Could you check a few things on this drawing? It's one solid part, dimensions in mm from its lowest x, y, z. A direction names the side the tool comes from. Give positions to 0.01 mm unless a question says otherwise; leave off trailing zeros. Write each loop counter-clockwise with the first axis right and the second up, starting at its lowest first coordinate (ties: lowest second). Pieces come first, ordered by that corner, then holes. Notation, with made-up numbers: (-1, 69.5) -> (26, 69.5) arc R23 ccw to (26, 78.5) -> close; hole circle Ø7 at (-25.5, 29). An arc over 180 degrees is marked (long way). Answer as CSV lines item,"result". Start each with the question number.
1. If we mould it in two halves opening along X, with no side actions, what happens to the marked faces 3, 4 and 5? For each: pulls with the +X half, pulls with the -X half, needs draft (parallel to the pull), parting line crosses it, or undercut.
2. I need wall thicknesses on line 1 (Y direction, x = 4.95, z = 11.15); line 2 (Z direction, x = 5.5, y = 3); line 3 (Z direction, x = 4.75, y = 2). Which ranges of each line are inside material? Lowest first, please. Write a range as [from, to].
3. If we section it at A-A on x = 4.95: Write out the boundary of the cut face in (y, z).
4. If we section it at D-D on y = 7.75: Write out the boundary of the cut face in (x, z).
5. On a 3-axis mill with a long thin cutter (end or side, diameter ignored), from which of +Z, -Z, +X, -X, +Y, -Y can I reach the whole of each face in a straight line? I mean the marked faces 1 and 2. Say none if no direction works.
6. I'm going to push flat-ended pins straight in: P1, Ø1.8, axis at x = 1.45, y = 4.95, coming from the +Z side; P2, Ø2, axis at y = 8, z = 3, coming from the -X side; P3, Ø2, axis at x = 2, z = 6, coming from the -Y side. Where does each tip first touch, or does it pass through?
7. If we section it at C-C on z = 14: Write out the boundary of the cut face in (x, y).
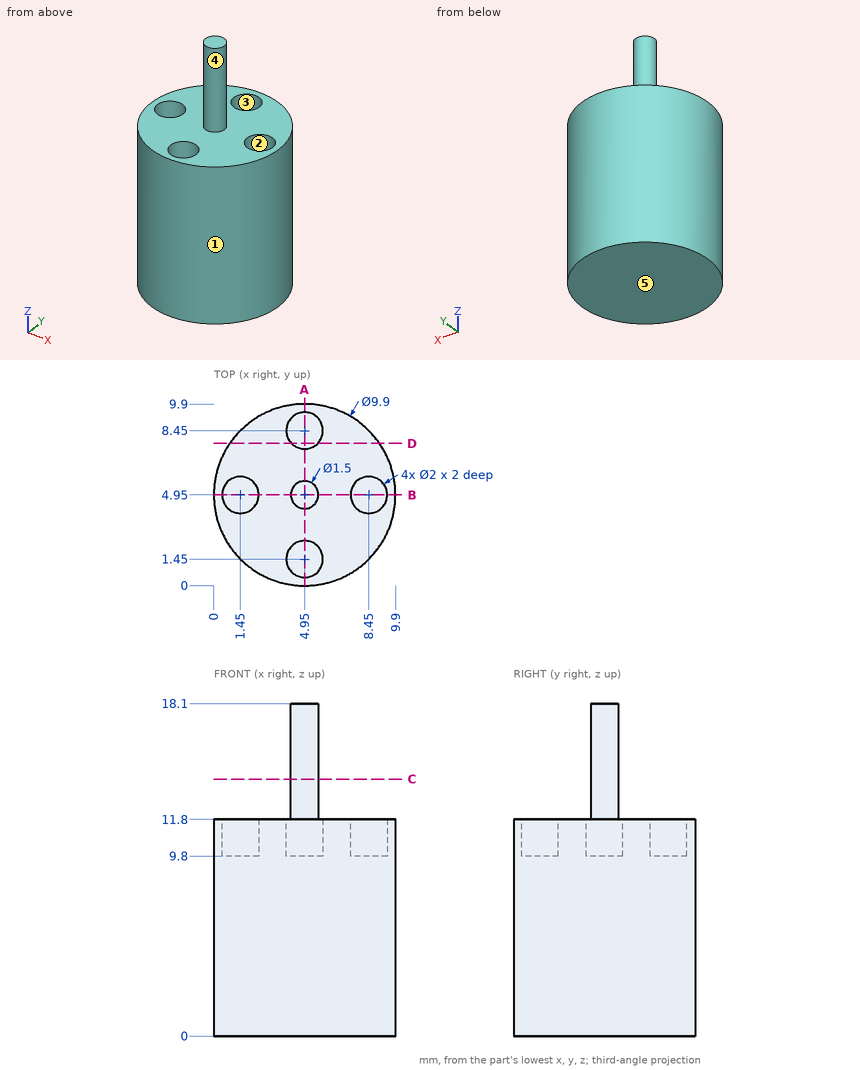
Computed values:
1,face 3,"undercut"
1,face 4,"parting line crosses it"
1,face 5,"needs draft"
2,line 1,"y = [0, 0.45], [2.45, 7.45], [9.45, 9.9]"
2,line 2,"z = [0, 11.8]"
2,line 3,"z = [0, 9.8]"
3,outline,"(0, 0) -> (9.9, 0) -> (9.9, 11.8) -> (9.45, 11.8) -> (9.45, 9.8) -> (7.45, 9.8) -> (7.45, 11.8) -> (5.7, 11.8) -> (5.7, 18.1) -> (4.2, 18.1) -> (4.2, 11.8) -> (2.45, 11.8) -> (2.45, 9.8) -> (0.45, 9.8) -> (0.45, 11.8) -> (0, 11.8) -> close"
4,outline,"(0.87, 0) -> (9.03, 0) -> (9.03, 11.8) -> (5.66, 11.8) -> (5.66, 9.8) -> (4.24, 9.8) -> (4.24, 11.8) -> (0.87, 11.8) -> close"
5,face 1,"+Z, -Z"
5,face 2,"+Z"
6,P1,"stops at z = 9.8"
6,P2,"stops at x = 0.44"
6,P3,"stops at y = 0.4"
7,outline,"circle Ø1.5 at (4.95, 4.95)"
